CAD build for the part. Positions are in the model's coordinates, mm. A direction names the side the tool comes from. Coordinates: 2 decimals unless noted, no trailing zeros. Loops run counter-clockwise (first coordinate to the right, second up) from the corner with the lowest first, then second, coordinate; pieces in that order, holes last. Notation, with made-up numbers: (67, -11.75) -> (89, -11.75) arc R9 ccw to (89, -5.75) -> close; hole circle Ø1 at (81, -36.5). An arc over 180 degrees is marked (long way). Answer as CSV lines item,"result". Start each with the question number.
```python
from build123d import *

# Parameters (mm, degrees)
F1_DEPTH  = 12.7
F4_DEPTH  = 3.81
F6_DEPTH  = 8.636
F8_DEPTH  = 29.211
F9_R      = 2.667
F10_DEPTH = 4.318
F12_DEPTH = 5.08
F13_R     = 1.7145
F14_DEPTH = 12.7
F15_R     = 5.715
F16_DEPTH = 2.794
F17_W     = 29.21
F17_H     = 12.7
F18_DEPTH = 10.668
F19_R     = 0.2


with BuildPart() as f1:
    # F0 (on Front) → F1 (new body)
    with BuildSketch(Plane.XZ):
        Polygon((-14.605, -3.7465), (14.605, -3.7465), (14.605, 3.7465), (14.605, 18.3515), (-14.605, 18.3515), (-14.605, 3.7465), align=None)
    extrude(amount=F1_DEPTH)

    # F3 (on offset) → F4 (cut)
    with BuildSketch(Plane.XZ.offset(6.35)):
        with BuildLine():
            Line((-9.144, -3.7465), (9.144, -3.7465))
            Line((9.144, -3.7465), (9.144, 6.9215))
            ThreePointArc((9.144, 6.9215), (0, 16.0655), (-9.144, 6.9215))
            Line((-9.144, 6.9215), (-9.144, -3.7465))
        make_face()
    extrude(amount=F4_DEPTH, mode=Mode.SUBTRACT)

    # F5 (on face) → F6 (cut)
    with BuildSketch(Plane.XZ.offset(12.7)):
        with BuildLine():
            Line((6.35, -3.7465), (4.8460111432, 5.3975))
            ThreePointArc((4.8460111432, 5.3975), (0, 12.0015), (-4.8460111432, 5.3975))
            Line((-4.8460111432, 5.3975), (-6.35, -3.7465))
            Line((-6.35, -3.7465), (6.35, -3.7465))
        make_face()
    extrude(amount=-F6_DEPTH, mode=Mode.SUBTRACT)

    # F7 (on face) → F8 (cut, through all)
    with BuildSketch(Plane.YZ.offset(14.605)):
        Polygon((-2.032, -0.6985), (0, -1.7145), (0, 16.3195), (-2.032, 15.3035), align=None)
    extrude(amount=-F8_DEPTH, mode=Mode.SUBTRACT)

    # F9 (on face) → F10 (cut, through all)
    with BuildSketch(Plane(origin=(0, -2.032, 0), x_dir=(-1, 0, 0), z_dir=(0, 1, 0))):
        with Locations((0, 6.9215)):
            Circle(F9_R)
    extrude(amount=-F10_DEPTH, mode=Mode.SUBTRACT)

    # F11 (on face) → F12 (cut)
    with BuildSketch(Plane.XY.offset(18.3515)):
        with BuildLine():
            Line((14.605, -4.191), (11.43, -4.191))
            ThreePointArc((11.43, -4.191), (8.255, -7.366), (11.43, -10.541))
            Line((11.43, -10.541), (14.605, -10.541))
            Line((14.605, -10.541), (14.605, -4.191))
        make_face()
        with BuildLine():
            ThreePointArc((-11.43, -10.541), (-8.255, -7.366), (-11.43, -4.191))
            Line((-11.43, -4.191), (-14.605, -4.191))
            Line((-14.605, -4.191), (-14.605, -10.541))
            Line((-14.605, -10.541), (-11.43, -10.541))
        make_face()
    extrude(amount=-F12_DEPTH, mode=Mode.SUBTRACT)

    # F13 (on face) → F14 (cut)
    with BuildSketch(Plane.XY.offset(13.2715)):
        with Locations((11.43, -7.366)):
            Circle(F13_R)
        with Locations((-11.43, -7.366)):
            Circle(F13_R)
    extrude(amount=-F14_DEPTH, mode=Mode.SUBTRACT)

    # F15 (on face) → F16 (cut)
    with BuildSketch(Plane.XZ.offset(6.35)):
        with Locations((0, 6.9215)):
            Circle(F15_R)
    extrude(amount=-F16_DEPTH, mode=Mode.SUBTRACT)

    # F17 (on face) → F18 (cut)
    with BuildSketch(Plane(origin=(0, 0, -3.7465), x_dir=(1, 0, 0), z_dir=(0, 0, -1))):
        with Locations((0, 6.35)):
            Rectangle(F17_W, F17_H)
    extrude(amount=-F18_DEPTH, mode=Mode.SUBTRACT)

    # F19
    f19_edges = [f1.edges().sort_by_distance(p)[0] for p in [
        (14.605, -12.7, 12.6365),
        (14.605, -2.032, 11.1125),
        (14.605, -1.016, 15.8115),
        (14.605, 0, 17.3355),
        (14.605, -10.541, 15.8115),
        (14.605, -4.191, 15.8115),
        (-14.605, -12.7, 12.6365),
        (-14.605, -10.541, 15.8115),
        (-14.605, -4.191, 15.8115),
        (-14.605, 0, 17.3355),
        (-14.605, -2.032, 11.1125),
        (-14.605, -1.016, 15.8115),
        (0, -12.7, 12.0015),
        (0, -10.16, 12.0015),
        (0, -6.35, 12.6365),
        (0, -3.556, 9.5885),
        (0, -2.032, 9.5885),
    ]]
    fillet(f19_edges, radius=F19_R)


solid = f1.part
```
Q1. Saw through at C-C (x = 12). List the corners of the cut face in (y, z), and give its area (3 significant figures).
Q2. Saw through at A-A (y = -8.5). List the corners of the cut face in (x, z) (1 decimal).
Q3. Two-plate mould, pull along Y, no slides. Class faces 4 (the cylindrical face through (-14.545, -1.112, 15.827)), 5 (the flat face through (-14.605, -8, 11)), 6 (the cylindrical face through (11.06, -9.04, 10.14)): pulls with the +Y half, pulls with the -Y half, needs draft (parallel to the pull), parting line crosses it, or undercut.
Q4. Saw through at B-B (x = 0). List the corners of the cut face in (y, z).
Q5. Probe probe 1 along Y at (x, z) = (11.43, 9.5); probe 2 along X at (y, z) = (-7.75, 12.25) (3 decimals); probe 3 along Y at (x, z) = (-4, 14.25). List the from-to ranges inside material, lowest first. Write a range as from..to.
Q6. Which spindle directions (+Z, -Z, +X, -X, +Y, -Y) get a long thin tool onto all of the face, cutting with end or side? Do faces 1 (the flat face through (13, -10.541, 16)), 2 (the flat face through (-13, -4.191, 16)), 3 (the flat face through (0, -10.16, 13)). Say none if no direction does.
Q7. Pin check, flat tips, straight feed: pin 1 Ø4 at (x, y) = (-10.5, -5.5) entering from +Z; pin 2 Ø1.9 at (x, y) = (12.5, -7.5) entering from +Z; pin 3 Ø2.5 at (x, y) = (11.43, -7.366) entering from -Z; pin 4 Ø1.7 at (x, z) = (2, 10) entering from -Y. Stop position of each tip, or through.
Q8. Saw through at D-D (z = 13.75). List the corners of the cut face in (x, y) (3 decimals).
Ans:
1,outline,"(-12.7, 6.92) -> (-8.98, 6.92) -> (-8.98, 13.27) -> (-10.54, 13.27) -> (-10.54, 18.35) -> (-12.7, 18.35) -> close; (-5.75, 6.92) -> (-2.03, 6.92) -> (-2.03, 15.3) -> (0, 16.32) -> (0, 18.35) -> (-4.19, 18.35) -> (-4.19, 13.27) -> (-5.75, 13.27) -> close"
1,area,"74.3 mm²"
2,outline,"(-14.6, 6.9) -> (-12.7, 6.9) -> (-12.7, 13.3) -> (-14.6, 13.3) -> close; (-10.1, 6.9) -> (-9.1, 6.9) arc R9.1 cw to (9.1, 6.9) -> (10.1, 6.9) -> (10.1, 13.3) -> (8.5, 13.3) -> (8.5, 18.4) -> (-8.5, 18.4) -> (-8.5, 13.3) -> (-10.1, 13.3) -> close; (12.7, 6.9) -> (14.6, 6.9) -> (14.6, 13.3) -> (12.7, 13.3) -> close"
3,face 4,"pulls with the +Y half"
3,face 5,"needs draft"
3,face 6,"undercut"
4,outline,"(-12.7, 12.2) arc R0.2 ccw to (-12.5, 12) -> (-10.36, 12) arc R0.2 ccw to (-10.16, 12.2) -> (-10.16, 16.07) -> (-6.35, 16.07) -> (-6.35, 12.84) arc R0.2 ccw to (-6.15, 12.64) -> (-3.56, 12.64) -> (-3.56, 9.79) arc R0.2 ccw to (-3.36, 9.59) -> (-2.23, 9.59) arc R0.2 ccw to (-2.03, 9.79) -> (-2.03, 15.3) -> (0, 16.32) -> (0, 18.35) -> (-12.7, 18.35) -> close"
5,probe 1,"y = -12.7..-9.08, -5.65..-2.03"
5,probe 2,"x = -14.605..-13.101, -9.759..-7.431, 7.431..9.759, 13.101..14.605"
5,probe 3,"y = -12.7..-10.16, -6.35..-2.03"
6,face 1,"+Z, +X"
6,face 2,"+Z, -X"
6,face 3,"-Z"
7,pin 1,"stops at z = 18.35"
7,pin 2,"stops at z = 13.27"
7,pin 3,"passes through"
7,pin 4,"stops at y = -3.56"
8,outline,"(-14.605, -12.5) arc R0.2 ccw to (-14.405, -12.7) -> (14.405, -12.7) arc R0.2 ccw to (14.605, -12.5) -> (14.605, -10.741) arc R0.2 ccw to (14.405, -10.541) -> (11.43, -10.541) arc R3.175 cw to (11.43, -4.191) -> (14.405, -4.191) arc R0.2 ccw to (14.605, -3.991) -> (14.605, -2.232) arc R0.2 ccw to (14.405, -2.032) -> (-14.405, -2.032) arc R0.2 ccw to (-14.605, -2.232) -> (-14.605, -3.991) arc R0.2 ccw to (-14.405, -4.191) -> (-11.43, -4.191) arc R3.175 cw to (-11.43, -10.541) -> (-14.405, -10.541) arc R0.2 ccw to (-14.605, -10.741) -> close; hole (-6.081, -10.16) -> (6.081, -10.16) -> (6.081, -6.35) -> (-6.081, -6.35) -> close"
